from build123d import *

# Parameters (mm, degrees)
EXTRUDE_1_DEPTH     = 3
SKETCH_2_R          = 21.5
CUT_EXTRUDE_1_DEPTH = 3
SKETCH_3_R          = 1.525
CUT_EXTRUDE_2_DEPTH = 3
SKETCH_4_W          = 38
SKETCH_4_H          = 60
SKETCH_4_R          = 1.6
EXTRUDE_2_DEPTH     = 3
SKETCH_13_R         = 1.525
CUT_EXTRUDE_7_DEPTH = 10
SKETCH_15_W         = 13
SKETCH_15_H         = 16
CUT_EXTRUDE_8_DEPTH = 10
FILLET_2_R          = 2
FILLET_3_R          = 1.5
SKETCH_16_R         = 2.1
CUT_EXTRUDE_9_DEPTH = 3
SKETCH_11_R         = 1.6
CUT_EXTRUDE_5_DEPTH = 10
CUT_EXTRUDE_START   = -10
CUT_EXTRUDE_3_DEPTH = 10
FILLET_1_R          = 10


with BuildPart() as part:
    # 草图1 → 凸台-拉伸1 (new body)
    with BuildSketch(Plane.XY):
        with BuildLine():
            Line((-19, -30), (19, -30))
            Line((19, -30), (26.093362093, -8.682537341))
            ThreePointArc((26.093362093, -8.682537341), (0, 27.5), (-26.093362093, -8.682537341))
            Line((-26.093362093, -8.682537341), (-19, -30))
        make_face()
    extrude(amount=EXTRUDE_1_DEPTH)

    # 草图2 → 切除-拉伸1 (cut)
    with BuildSketch(Plane.XY.offset(3)):
        Circle(SKETCH_2_R)
    extrude(amount=-CUT_EXTRUDE_1_DEPTH, mode=Mode.SUBTRACT)

    # 草图3 → 切除-拉伸2 (cut)
    with BuildSketch(Plane.XY.offset(3)):
        with Locations((17.324116139, 17.324116139)):
            Circle(SKETCH_3_R)
        with Locations((24.5, 0)):
            Circle(SKETCH_3_R)
        with Locations((17.324116139, -17.324116139)):
            Circle(SKETCH_3_R)
        with Locations((0, -24.5)):
            Circle(SKETCH_3_R)
        with Locations((-17.324116139, -17.324116139)):
            Circle(SKETCH_3_R)
        with Locations((-24.5, 0)):
            Circle(SKETCH_3_R)
        with Locations((-17.324116139, 17.324116139)):
            Circle(SKETCH_3_R)
        with Locations((0, 24.5)):
            Circle(SKETCH_3_R)
    extrude(amount=-CUT_EXTRUDE_2_DEPTH, mode=Mode.SUBTRACT)

    # 草图4 → 凸台-拉伸2 (add)
    with BuildSketch(Plane.XY.offset(3)):
        with Locations((0, -60)):
            Rectangle(SKETCH_4_W, SKETCH_4_H)
        with Locations((-12.5, -84)):
            Circle(SKETCH_4_R, mode=Mode.SUBTRACT)
        with Locations((12.5, -84)):
            Circle(SKETCH_4_R, mode=Mode.SUBTRACT)
    extrude(amount=-EXTRUDE_2_DEPTH)

    # 草图13 → 切除-拉伸7 (cut)
    with BuildSketch(Plane(origin=(0, 0, 0), x_dir=(-1, 0, 0), z_dir=(0, 0, -1))):
        with Locations((16, -73)):
            Circle(SKETCH_13_R)
        with Locations((16, -53)):
            Circle(SKETCH_13_R)
        with Locations((-16, -53)):
            Circle(SKETCH_13_R)
        with Locations((-16, -73)):
            Circle(SKETCH_13_R)
    extrude(amount=-CUT_EXTRUDE_7_DEPTH, mode=Mode.SUBTRACT)

    # 草图15 → 切除-拉伸8 (cut)
    with BuildSketch(Plane(origin=(0, 0, 0), x_dir=(-1, 0, 0), z_dir=(0, 0, -1))):
        with Locations((-9.5, -40)):
            Rectangle(SKETCH_15_W, SKETCH_15_H)
        with Locations((9.5, -40)):
            Rectangle(SKETCH_15_W, SKETCH_15_H)
        Polygon((7.283009434, -55.5), (-7.283009434, -55.5), (0, -60.051880896), align=None)
        Polygon((-4.716990566, -63), (-13.5, -57.510619104), (-13.5, -68.489380896), align=None)
        Polygon((7.283009434, -70.5), (0, -65.948119104), (-7.283009434, -70.5), align=None)
        Polygon((13.5, -57.510619104), (4.716990566, -63), (13.5, -68.489380896), align=None)
    extrude(amount=-CUT_EXTRUDE_8_DEPTH, mode=Mode.SUBTRACT)

    # 圆角2
    fillet_2_edges = [part.edges().sort_by_distance(p)[0] for p in [
        (4.716990566, -63, 1.5),
        (0, -65.948119104, 1.5),
        (0, -60.051880896, 1.5),
        (-3, -32, 1.5),
        (-16, -32, 1.5),
        (-16, -48, 1.5),
        (-3, -48, 1.5),
        (-4.716990566, -63, 1.5),
        (16, -32, 1.5),
        (3, -32, 1.5),
        (3, -48, 1.5),
        (16, -48, 1.5),
    ]]
    fillet(fillet_2_edges, radius=FILLET_2_R)

    # 圆角3
    fillet_3_edges = [part.edges().sort_by_distance(p)[0] for p in [
        (13.5, -68.489380896, 1.5),
        (13.5, -57.510619104, 1.5),
        (7.283009434, -70.5, 1.5),
        (-7.283009434, -70.5, 1.5),
        (7.283009434, -55.5, 1.5),
        (-7.283009434, -55.5, 1.5),
        (-13.5, -68.489380896, 1.5),
        (-13.5, -57.510619104, 1.5),
    ]]
    fillet(fillet_3_edges, radius=FILLET_3_R)

    # 草图16 → 切除-拉伸9 (cut)
    with BuildSketch(Plane(origin=(0, 0, 0), x_dir=(-1, 0, 0), z_dir=(0, 0, -1))):
        with Locations((0, -63)):
            Circle(SKETCH_16_R)
    extrude(amount=-CUT_EXTRUDE_9_DEPTH, mode=Mode.SUBTRACT)

    # 草图11 → 切除-拉伸5 (cut)
    with BuildSketch(Plane.XY.offset(3)):
        with Locations((-12.5, -64)):
            Circle(SKETCH_11_R)
        with Locations((12.5, -64)):
            Circle(SKETCH_11_R)
    extrude(amount=-CUT_EXTRUDE_5_DEPTH, mode=Mode.SUBTRACT)

    # 草图5 → 切除-拉伸3 (cut)
    with BuildSketch(Plane.XY.offset(3).offset(CUT_EXTRUDE_START)):
        with BuildLine():
            ThreePointArc((8.797072002, -26.054971199), (10.594225082, -26.485562705), (11.598652136, -24.934339146))
            ThreePointArc((11.598652136, -24.934339146), (10.2132436, -25.533108999), (8.797072002, -26.054971199))
        make_face()
        with BuildLine():
            ThreePointArc((-8.797072002, -26.054971199), (-10.2132436, -25.533108999), (-11.598652136, -24.934339146))
            ThreePointArc((-11.598652136, -24.934339146), (-10.594225082, -26.485562705), (-8.797072002, -26.054971199))
        make_face()
    extrude(amount=CUT_EXTRUDE_3_DEPTH, mode=Mode.SUBTRACT)

    # 圆角1
    fillet_1_edges = [part.edges().sort_by_distance(p)[0] for p in [
        (19, -30, 1.5),
        (-19, -30, 1.5),
    ]]
    fillet(fillet_1_edges, radius=FILLET_1_R)


solid = part.part
Check sheet for the modelled part. Datum: model origin and axes. Units: mm. Give positions to 0.01 mm unless a question says otherwise; leave off trailing zeros. Write each loop counter-clockwise with the first axis right and the second up, starting at its lowest first coordinate (ties: lowest second). Pieces come first, ordered by that corner, then holes. Notation, with made-up numbers: M 51.5,32 L 78.5,32 A13 ccw 78.5,36 Z; hole C -10.5,-13.5 d10. An arc over 180 degrees is marked long. Use one line per item in the form item = value.
(1) Section check A-A on y = -73. Record the boundary of the cut face in (x, z) (3 decimals).
Answer block:
outline = M -19,0 L -17.525,0 L -17.525,3 L -19,3 Z; M -14.475,0 L 14.475,0 L 14.475,3 L -14.475,3 Z; M 17.525,0 L 19,0 L 19,3 L 17.525,3 Z
(2) Section check D-D on z = 1.65. State how many separate pieces and enclosed holes the cut face has, plus the area to 3 significant figures.
Answer block:
separate_pieces = 1
enclosed_holes = 24
area = 2,780 mm2
(3) Material ranges on line 1 along X through (y, z) = (-73, 1.9) (3 decimals); line 2 along X through (y, z) = (-37, 1.65); line 3 along X through (y, z) = (-62.5, 2.7), recorded low to high.
Answer block:
line_1 = -19 to -17.525, -14.475 to 14.475, 17.525 to 19
line_2 = -19 to -16, -3 to 3, 16 to 19
line_3 = -19 to -13.5, -6.55 to -2.04, 2.04 to 6.55, 13.5 to 19
(4) Section check C-C on y = 0. Record the boundary of the cut face in (x, z) (3 decimals), plus the area to 3 significant figures.
Answer block:
outline = M -27.5,0 L -26.025,0 L -26.025,3 L -27.5,3 Z; M -22.975,0 L -21.5,0 L -21.5,3 L -22.975,3 Z; M 21.5,0 L 22.975,0 L 22.975,3 L 21.5,3 Z; M 26.025,0 L 27.5,0 L 27.5,3 L 26.025,3 Z
area = 17.7 mm2
(5) Section check B-B on x = 0. Record the boundary of the cut face in (y, z) (3 decimals).
Answer block:
outline = M -90,0 L -70.5,0 L -70.5,3 L -90,3 Z; M -66.307,0 L -65.1,0 L -65.1,3 L -66.307,3 Z; M -60.9,0 L -59.693,0 L -59.693,3 L -60.9,3 Z; M -55.5,0 L -26.025,0 L -26.025,3 L -55.5,3 Z; M -22.975,0 L -21.5,0 L -21.5,3 L -22.975,3 Z; M 21.5,0 L 22.975,0 L 22.975,3 L 21.5,3 Z; M 26.025,0 L 27.5,0 L 27.5,3 L 26.025,3 Z
(6) Draft check along X on faces 1 (the flat face through (-22.85, -18.43, 1.48)), 2 (the flat face through (19, -61, 2)), 3 (the cylindrical face through (12.708, -58.894, 1.521)), 4 (the flat face through (0, -90, 2)). Enter one of: pulls with the +X half, pulls with the -X half, needs draft (parallel to the pull), parting line crosses it, or undercut.
Answer block:
face_1 = pulls with the -X half
face_2 = pulls with the +X half
face_3 = undercut
face_4 = needs draft
(7) Depth check by flat-ended pin: P1, Ø1.5, axis at y = -48, z = 2.5, coming from the +X side; P2, Ø2, axis at x = 2, y = -67.5, coming from the +Z side; P3, Ø4, axis at x = 0, y = -63, coming from the +Z side (3 decimals); P4, Ø0.9, axis at y = -67, z = 1, coming from the -X side. Enter the tip coordinate at first touch or a pass-through.
Answer block:
P1 = 19
P2 = 3
P3 = through
P4 = -19
